Autodesk Inventor part; units mm, degrees
ref_plane "Work Plane1" through (29, 0, 0) normal (0, -1, 0) x (1, 0, 0)
ref_plane "YZ Plane" through (0, 0, 0) normal (1, 0, 0) x (0, 1, 0)
ref_plane "XZ Plane" through (0, 0, 0) normal (0, 1, 0) x (-1, 0, 0)
sketch "Sketch1" plane through (0, 0, 0) normal (0, 0, 1) x (1, 0, 0)
  line L0 (-1.1667, 0) -> (60, 0)
  line L1 (60, 0) -> (60, 2.5)
  line L2 (60, 2.5) -> (38, 2.5)
  line L3 (38, 2.5) -> (37.5091, 2.5)
  line L4 (37.5091, 2.5) -> (0, 2.5)
  line L5 (0, 2.5) -> (0, 4.25)
  line L6 (0, 4.25) -> (-5, 4.25)
  line L7 (-5, 4.25) -> (-5, 2.3094)
  line L8 (-5, 2.3094) -> (-2.5, 2.3094)
  line L9 (-2.5, 2.3094) -> (-1.1667, 0)
  line L10 (-22, 0) -> (97, 0)
  line L11 (0, -0.85) -> (0, 5.1)
  line L12 (38, 2.5) -> (0, 2.5) construction
  dimension "d1" = 22
  dimension "d2" = 0.4909
  dimension "d3" = 5
  dimension "d4" = 2.5
  dimension "d5" = 60
  dimension "d6" = 5
  dimension "d7" = 5
  dimension "d8" = 4.6188
  dimension "d9" = 8.5
  dimension "d26" = 60
revolve "Body" add sketch "Sketch1" angle 360 about axis through (-1.1667, 0, 0) along (1, 0, 0)
sketch "Sketch2" plane through (-5, 0, 0) normal (-1, 0, 0) x (0, 0, 1)
  circle A0 centre (0, 0) radius 2.3094
  line L0 (0, -5.95) -> (0, 5.95)
  line L1 (-5.95, 0) -> (5.95, 0)
  line L2 (2.3094, 0) -> (1.1547, -2)
  line L3 (1.1547, -2) -> (-1.1547, -2)
  line L4 (-1.1547, -2) -> (-2.3094, 0)
  line L5 (-2.3094, 0) -> (-1.1547, 2)
  line L6 (-1.1547, 2) -> (1.1547, 2)
  line L7 (1.1547, 2) -> (2.3094, 0)
extrude "Slot" add sketch "Sketch2" against normal up to next contours L7 A0 | A0 L2 | L6 L0 A0 | A0 L0 L3 | L0 L6 A0 | A0 L3 L0 | L4 A0 | A0 L5
fillet "Fillet1" radius 0.5 1 edges at (-5, -4.25, 0)
thread "Thread"
chamfer "Chamfer1" distance 0.4908 distance2 0.4908 1 edges at (60, -2.5, 0) measured on face at (60, -0.6238, -0.819)
ref_plane "Work Plane1" through (29, 0, 0) normal (0, -1, 0) x (1, 0, 0)
fillet "Fillet2" radius 0.2 1 edges at (0, -2.5, 0)
equation "\"d30\" = R"
equation "\"d17\" = RR"
equation "\"d13\" = GEL"
equation "\"d15\" = -0.5 * SPD + 0.5 * GD"
equation "\"d16\" = GUL"
equation "\"d1\" = GEL"
equation "\"d3\" = KOH"
equation "\"d4\" = INTI"
equation "\"d6\" = GD"
equation "\"d7\" = BDM"
equation "\"d8\" = 1.1547 * SW"
equation "\"d9\" = KOD"
equation "\"d26\" = NLG"
equation "\"GD\" = NND"
equation "\"NLG\" = 60"
equation "\"GEL\" = 22"
equation "\"KOD\" = 8.5"
equation "\"KOH\" = 5"
equation "\"INTI\" = 2.5"
equation "\"GAL\" = 0.61345 * PTC"
equation "\"GUL\" = 0.61345 * PTC"
equation "\"BDM\" = NND"
equation "\"SW\" = 4"
equation "\"RR\" = 0.5"
equation "\"SPD\" = NND - 1.2269 * PTC"
equation "\"R\" = 0.2"
equation "\"TOA\" = 30deg"
equation "\"GD1\" = THREADDIA - 1.2269 * PTC"
equation "\"THREADDIA\" = 5"
equation "\"FAWI\" = 45deg"
equation "\"ANG\" = 120deg"
equation "\"PTC\" = 0.8"
equation "\"NND\" = 5"
equation "\"E0\" = 1.155 * SW"
properties material "Steel, Mild"
The model under review builds one solid part; all positions refer to its coordinate system, in mm. A direction names the side the tool comes from. Round coordinates to 2 decimals unless told otherwise and drop trailing zeros. Loops run counter-clockwise (first coordinate to the right, second up) from the corner with the lowest first, then second, coordinate; pieces in that order, holes last. Notation, with made-up numbers: (87.5, 73.5) - (96.5, 73.5) arc R15 ccw to (96.5, 77.5) - close; hole circle Ø7 at (49.5, -20.75). An arc over 180 degrees is marked (long way). Write each question's results on one line, items separated by ' | '. Start each with the question number.
Q1. Draft analysis for pull direction Y (two halves, no side actions). For faces 1 (the cylindrical face through (29.44, -0.54, 2.44)), 2 (the flat face through (-4, -2, 0)), 3 (the flat face through (-5, -2, 2)), state which applies: pulls with the +Y half, pulls with the -Y half, needs draft (parallel to the pull), parting line crosses it, or undercut.
Q2. Wall thickness on line 1 along X through (y, z) = (-1, 2.75); line 2 along Y through (x, z) = (0.5, 1.5): over which ranges is each line inside the solid? List them lowest first. Write a range as [from, to].
Q3. Insertion check: P1, Ø2, axis at x = 13, z = 0, coming from the -Y side; P2, Ø1, axis at x = 8, y = 1.5, coming from the +Z side; P3, Ø1.5, axis at x = 15.5, z = -1.5, coming from the +Y side. Each pin has a flat end and moves straight along its axis. Give the tip position at first contact, or say it passes through.
Q4. Take a section at A-A on x = 7.5. Give the boundary of the cut face in (y, z).
Q5. Tool access review of faces 4 (the cylindrical face through (-2.282, 2.285, -3.584)), 5 (the flat face through (0, 0, -3)), 6 (the flat face through (-3.679, -1.014, -1.724)): name each direction out of +Z, -Z, +X, -X, +Y, -Y from which nothing blocks a thin tool from reaching the whole face with its end or side.
Data:
1) face 1: parting line crosses it | face 2: undercut | face 3: needs draft
2) line 1: x = [-5, 0] | line 2: y = [-2, 2]
3) P1: stops at y = -2.5 | P2: stops at z = 2.29 | P3: stops at y = 2.38
4) outline: circle Ø5 at (0, 0)
5) face 4: +X, -X | face 5: +X | face 6: -X
